```python
from build123d import *

# Parameters (mm, degrees)
F0_R     = 0.9
F1_DEPTH = 45
F2_DEPTH = 5
F3_DEPTH = 1
F4_R     = 5.995213452
F5_DEPTH = 25


with BuildPart() as f1:
    # F0 (on Top) → F1 (new body)
    with BuildSketch(Plane.XY):
        with BuildLine():
            Line((69.6141044706, -60.8155948031), (92.0655032996, 8.2827057594))
            ThreePointArc((92.0655032996, 8.2827057594), (92.0655032996, 29.9138953656), (79.3510090595, 47.4138953656))
            Line((79.3510090595, 47.4138953656), (20.5724838302, 90.1189936781))
            ThreePointArc((20.5724838302, 90.1189936781), (0, 96.803398875), (-20.5724838302, 90.1189936781))
            Line((-20.5724838302, 90.1189936781), (-79.3510090595, 47.4138953656))
            ThreePointArc((-79.3510090595, 47.4138953656), (-92.0655032996, 29.9138953656), (-92.0655032996, 8.2827057594))
            Line((-92.0655032996, 8.2827057594), (-69.6141044706, -60.8155948031))
            ThreePointArc((-69.6141044706, -60.8155948031), (-56.8996102305, -78.3155948031), (-36.3271264003, -85))
            Line((-36.3271264003, -85), (-35.7632361451, -82))
            Line((-35.7632361451, -82), (-36.3271264003, -82))
            ThreePointArc((-36.3271264003, -82), (-38.5650226814, -81.9216512768), (-40.7919604428, -81.6869887647))
            ThreePointArc((-40.7919604428, -81.6869887647), (-56.9006983727, -74.5097559412), (-66.7609349217, -59.88854382))
            Line((-66.7609349217, -59.88854382), (-89.2123337507, 9.2097567425))
            ThreePointArc((-89.2123337507, 9.2097567425), (-89.2123337507, 28.9868443825), (-77.5876533026, 44.9868443825))
            Line((-77.5876533026, 44.9868443825), (-18.8091280734, 87.691942695))
            ThreePointArc((-18.8091280734, 87.691942695), (0, 93.803398875), (18.8091280734, 87.691942695))
            Line((18.8091280734, 87.691942695), (77.5876533026, 44.9868443825))
            ThreePointArc((77.5876533026, 44.9868443825), (89.2123337507, 28.9868443825), (89.2123337507, 9.2097567425))
            Line((89.2123337507, 9.2097567425), (66.7609349217, -59.88854382))
            ThreePointArc((66.7609349217, -59.88854382), (56.9006983727, -74.5097559412), (40.7919604428, -81.6869887647))
            ThreePointArc((40.7919604428, -81.6869887647), (38.5650226814, -81.9216512768), (36.3271264003, -82))
            Line((36.3271264003, -82), (35.7632361451, -82))
            Line((35.7632361451, -82), (36.3271264003, -85))
            ThreePointArc((36.3271264003, -85), (56.8996102305, -78.3155948031), (69.6141044706, -60.8155948031))
        make_face()
        with Locations((79.0327965041, -25.6793122326)):
            Circle(F0_R, mode=Mode.SUBTRACT)
        with Locations((-90.2584959186, 29.3267630763)):
            Circle(F0_R, mode=Mode.SUBTRACT)
    extrude(amount=F1_DEPTH)

    # F0 (on Top) → F2 (join)
    with BuildSketch(Plane.XY):
        with BuildLine():
            Line((19.6557918633, 3.6945698296), (34.8234190532, -77))
            Line((34.8234190532, -77), (36.3271264003, -77))
            ThreePointArc((36.3271264003, -77), (38.1009794725, -76.9416674554), (39.8671678511, -76.7669218725))
            Line((39.8671678511, -76.7669218725), (24.5697398292, 4.618212287))
            ThreePointArc((24.5697398292, 4.618212287), (0, 25), (-24.5697398292, 4.618212287))
            Line((-24.5697398292, 4.618212287), (-39.8671678511, -76.7669218725))
            ThreePointArc((-39.8671678511, -76.7669218725), (-38.1009794725, -76.9416674554), (-36.3271264003, -77))
            Line((-36.3271264003, -77), (-34.8234190532, -77))
            Line((-34.8234190532, -77), (-19.6557918633, 3.6945698296))
            ThreePointArc((-19.6557918633, 3.6945698296), (0, 20), (19.6557918633, 3.6945698296))
        make_face()
        with BuildLine():
            Line((-36.3271264003, -82), (-35.7632361451, -82))
            Line((-35.7632361451, -82), (-34.8234190532, -77))
            Line((-34.8234190532, -77), (-36.3271264003, -77))
            ThreePointArc((-36.3271264003, -77), (-38.1009794725, -76.9416674554), (-39.8671678511, -76.7669218725))
            Line((-39.8671678511, -76.7669218725), (-40.7919604428, -81.6869887647))
            ThreePointArc((-40.7919604428, -81.6869887647), (-38.5650226814, -81.9216512768), (-36.3271264003, -82))
        make_face()
        with BuildLine():
            Line((34.8234190532, -77), (35.7632361451, -82))
            Line((35.7632361451, -82), (36.3271264003, -82))
            ThreePointArc((36.3271264003, -82), (38.5650226814, -81.9216512768), (40.7919604428, -81.6869887647))
            Line((40.7919604428, -81.6869887647), (39.8671678511, -76.7669218725))
            ThreePointArc((39.8671678511, -76.7669218725), (38.1009794725, -76.9416674554), (36.3271264003, -77))
            Line((36.3271264003, -77), (34.8234190532, -77))
        make_face()
    extrude(amount=F2_DEPTH)

    # F0 (on Top) → F3 (join)
    with BuildSketch(Plane.XY):
        Polygon((-35.7632361451, -82), (35.7632361451, -82), (34.8234190532, -77), (-34.8234190532, -77), align=None)
        Polygon((-36.3271264003, -85), (36.3271264003, -85), (35.7632361451, -82), (-35.7632361451, -82), align=None)
        with BuildLine():
            Line((-34.8234190532, -77), (34.8234190532, -77))
            Line((34.8234190532, -77), (19.6557918633, 3.6945698296))
            ThreePointArc((19.6557918633, 3.6945698296), (0, 20), (-19.6557918633, 3.6945698296))
            Line((-19.6557918633, 3.6945698296), (-34.8234190532, -77))
        make_face()
        with BuildLine():
            Line((39.8671678511, -76.7669218725), (40.7919604428, -81.6869887647))
            ThreePointArc((40.7919604428, -81.6869887647), (56.9006983727, -74.5097559412), (66.7609349217, -59.88854382))
            Line((66.7609349217, -59.88854382), (89.2123337507, 9.2097567425))
            ThreePointArc((89.2123337507, 9.2097567425), (89.2123337507, 28.9868443825), (77.5876533026, 44.9868443825))
            Line((77.5876533026, 44.9868443825), (18.8091280734, 87.691942695))
            ThreePointArc((18.8091280734, 87.691942695), (0, 93.803398875), (-18.8091280734, 87.691942695))
            Line((-18.8091280734, 87.691942695), (-77.5876533026, 44.9868443825))
            ThreePointArc((-77.5876533026, 44.9868443825), (-89.2123337507, 28.9868443825), (-89.2123337507, 9.2097567425))
            Line((-89.2123337507, 9.2097567425), (-66.7609349217, -59.88854382))
            ThreePointArc((-66.7609349217, -59.88854382), (-56.9006983727, -74.5097559412), (-40.7919604428, -81.6869887647))
            Line((-40.7919604428, -81.6869887647), (-39.8671678511, -76.7669218725))
            ThreePointArc((-39.8671678511, -76.7669218725), (-53.5981184837, -70.7536221526), (-62.0056523402, -58.3434588481))
            Line((-62.0056523402, -58.3434588481), (-84.4570511692, 10.7548417144))
            ThreePointArc((-84.4570511692, 10.7548417144), (-84.4570511692, 27.4417594106), (-74.6487270411, 40.9417594106))
            Line((-74.6487270411, 40.9417594106), (-15.8702018119, 83.6468577231))
            ThreePointArc((-15.8702018119, 83.6468577231), (0, 88.803398875), (15.8702018119, 83.6468577231))
            Line((15.8702018119, 83.6468577231), (74.6487270411, 40.9417594106))
            ThreePointArc((74.6487270411, 40.9417594106), (84.4570511692, 27.4417594106), (84.4570511692, 10.7548417144))
            Line((84.4570511692, 10.7548417144), (62.0056523402, -58.3434588481))
            ThreePointArc((62.0056523402, -58.3434588481), (53.5981184837, -70.7536221526), (39.8671678511, -76.7669218725))
        make_face()
    extrude(amount=F3_DEPTH)

    # F4 (on face) → F5 (cut)
    with BuildSketch(Plane(origin=(-80.8398038851, -26.2664445219, 0), x_dir=(0.3090169944, -0.9510565163, 0), z_dir=(-0.9510565163, -0.3090169944, 0))):
        with Locations((45.5608554184, 22.5)):
            Circle(F4_R)
    extrude(amount=-F5_DEPTH, mode=Mode.SUBTRACT)


solid = f1.part
```
Check sheet for the modelled part. Datum: model origin and axes. Units: mm. A direction names the side the tool comes from. Coordinates: 2 decimals unless noted, no trailing zeros. Order: outer loops, then holes, each group sorted by start corner. A loop starts at its lowest first (then second) coordinate and runs counter-clockwise, first axis right, second up. Notation, with made-up numbers: (-2.75, -37) -> (43.25, -37) arc R21 ccw to (43.25, -15) -> close; hole circle Ø3 at (71, 3.5). An arc over 180 degrees is marked (long way). Write each question's results on one line, items separated by ' | '. Start each with the question number.
1) Section check D-D (x = 4). Enter the section's corners in (y, z), and give its area (3 significant figures).
2) Section check C-C (z = 34.5). Enter the section's corners in (x, y), and give its area (3 significant figures).
3) Depth check by flat-ended pin: pin 1 (3 mm diameter, centred on y = -5.5, z = 16.5, fed in from +X); pin 2 (8 mm diameter, centred on x = 36, z = 16.5, fed in from +Y); pin 3 (2 mm diameter, centred on x = -42.5, z = 5, fed in from +Y). Enter the tip coordinate at first touch or a pass-through.
4) Section check A-A (y = -40.5). Enter the section's corners in (x, z), and give its area (3 significant figures).
5) Material ranges on line 1 along Z through (x, y) = (22, -19); line 2 along Y through (x, z) = (-47.5, 43.5) (3 decimals); line 3 along Y through (x, z) = (-55, 24.5), recorded low to high.
6) Draft check along Y on faces 4 (the face through (-91.969, 30.206, 22.185)), 5 (the face through (-1, -43, 1)), 6 (the face through (-45.671, 61.995, 0.493)), 7 (the face through (56.65, -78.495, 22.185)). Enter one of: pulls with the +Y half, pulls with the -Y half, needs draft (parallel to the pull), parting line crosses it, or undercut.
7) Set-up check for faces 1 (the face through (-61.762, -73.796, 20.204)), 2 (the face through (-77.83, -25.82, 22.69)), 3 (the face through (-84.53, 27.22, 0.49)): record each of +Z, -Z, +X, -X, +Y, -Y from which the full face is reachable in a straight line by a thin tool's end or side.
8) Section check B-B (x = 29). Enter the section's corners in (y, z).
Checked values:
1) outline: (-85, 0) -> (24.68, 0) -> (24.68, 5) -> (19.6, 5) -> (19.6, 1) -> (-85, 1) -> close; (88.51, 0) -> (96.57, 0) -> (96.57, 45) -> (93.55, 45) -> (93.55, 1) -> (88.51, 1) -> close | area: 271 mm²
2) outline: (-92.07, 8.28) -> (-69.61, -60.82) arc R35 ccw to (-36.33, -85) -> (-35.76, -82) -> (-36.33, -82) arc R32 cw to (-66.76, -59.89) -> (-89.21, 9.21) arc R32 cw to (-77.59, 44.99) -> (-18.81, 87.69) arc R32 cw to (18.81, 87.69) -> (77.59, 44.99) arc R32 cw to (89.21, 9.21) -> (66.76, -59.89) arc R32 cw to (36.33, -82) -> (35.76, -82) -> (36.33, -85) arc R35 ccw to (69.61, -60.82) -> (92.07, 8.28) arc R35 ccw to (79.35, 47.41) -> (20.57, 90.12) arc R35 ccw to (-20.57, 90.12) -> (-79.35, 47.41) arc R35 ccw to start; hole circle Ø1.8 at (-90.26, 29.33); hole circle Ø1.8 at (79.03, -25.68) | area: 1,500 mm²
3) pin 1: x = 88.07 | pin 2: y = 81.82 | pin 3: y = 74.91
4) outline: (-76.22, 0) -> (-67.8, 0) -> (-67.8, 1) -> (-73.06, 1) -> (-73.06, 45) -> (-76.22, 45) -> close; (-33.05, 0) -> (33.05, 0) -> (33.05, 5) -> (27.96, 5) -> (27.96, 1) -> (-27.96, 1) -> (-27.96, 5) -> (-33.05, 5) -> close; (67.8, 0) -> (76.22, 0) -> (76.22, 45) -> (73.06, 45) -> (73.06, 1) -> (67.8, 1) -> close | area: 401 mm²
5) line 1: 0 to 1 | line 2: -83.169 to -79.986, 66.847 to 70.555 | line 3: -79.6 to -75.99, 61.4 to 65.11
6) face 4: parting line crosses it | face 5: needs draft | face 6: undercut | face 7: pulls with the -Y half
7) face 1: none | face 2: +Z | face 3: +Z, -Z
8) outline: (-85, 0) -> (-18.95, 0) -> (-18.95, 5) -> (-46.02, 5) -> (-46.02, 1) -> (-85, 1) -> close; (74.11, 0) -> (84, 0) -> (84, 45) -> (80.29, 45) -> (80.29, 1) -> (74.11, 1) -> close
